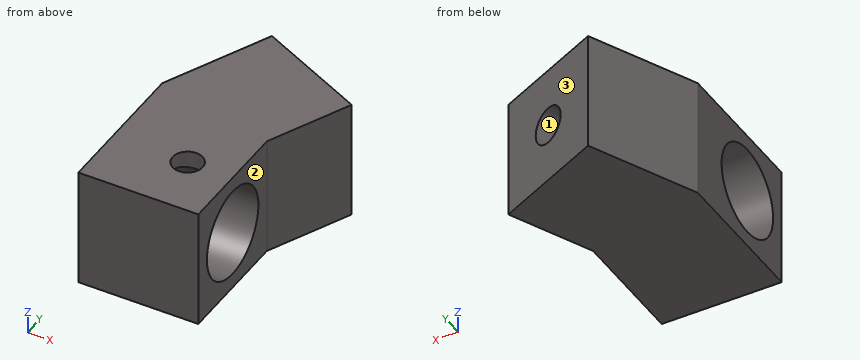
from build123d import *

# Parameters (mm, degrees)
BOSS_EXTRUDE1_DEPTH = 8
CUT_EXTRUDE1_REACH  = 10
SKETCH3_R           = 3
CUT_EXTRUDE2_REACH  = 10
SKETCH4_R           = 1
SKETCH5_R           = 1.25
CUT_EXTRUDE3_DEPTH  = 3


with BuildPart() as part:
    # Sketch2 → Boss-Extrude1 (new body)
    with BuildSketch(Plane.XY):
        Polygon((8, 0), (0, 0), (0, 9.773557301), (3.285247274, 16.818792816), (10.53570957, 13.437846722), (8, 8), align=None)
    extrude(amount=BOSS_EXTRUDE1_DEPTH)

    # Sketch3 → Cut-Extrude1 (cut, up to next)
    with BuildSketch(Plane(origin=(8, 0, 0), x_dir=(0, 0, -1), z_dir=(1, 0, 0)), mode=Mode.PRIVATE) as cut_extrude1_sk1:
        with Locations((-4, 4)):
            Circle(SKETCH3_R)
    cut_extrude1_tool1 = extrude(cut_extrude1_sk1.sketch, amount=-CUT_EXTRUDE1_REACH, mode=Mode.PRIVATE) & part.part
    add(cut_extrude1_tool1.solids().sort_by_distance((8, 4, 4))[0], mode=Mode.SUBTRACT)

    # Sketch4 → Cut-Extrude2 (cut, up to next)
    with BuildSketch(Plane.XY.offset(8), mode=Mode.PRIVATE) as cut_extrude2_sk1:
        with Locations((5, 4)):
            Circle(SKETCH4_R)
    cut_extrude2_tool1 = extrude(cut_extrude2_sk1.sketch, amount=-CUT_EXTRUDE2_REACH, mode=Mode.PRIVATE) & part.part
    add(cut_extrude2_tool1.solids().sort_by_distance((5, 4, 8))[0], mode=Mode.SUBTRACT)

    # Sketch5 → Cut-Extrude3 (cut)
    with BuildSketch(Plane(origin=(7.028736904, 15.073174933, 0), x_dir=(0.906307787, -0.422618262, 0), z_dir=(0.422618262, 0.906307787, 0))):
        with Locations((-0.130483798, -4)):
            Circle(SKETCH5_R)
    extrude(amount=-CUT_EXTRUDE3_DEPTH, mode=Mode.SUBTRACT)


solid = part.part
Work out the finished part from the listing and answer in its coordinate system (mm). Face numbers are marked on the shaded views. Coordinates: 2 decimals unless noted, no trailing zeros. Loops run counter-clockwise (first coordinate to the right, second up) from the corner with the lowest first, then second, coordinate; pieces in that order, holes last. Notation, with made-up numbers: M 5.25,51.5 L 51.25,51.5 A15 cw 51.25,74.5 Z; hole C 12.25,85.25 d8. An arc over 180 degrees is marked long. Answer in a Markdown table with one row per item. Add a question column.
1. Find section C-C, the plane y = 2. Write down the section's boundary in (x, z), then the cut area to 3 significant figures.
2. Find section D-D, the plane z = 5.5. Write down the section's boundary in (x, y), then the cut area to 3 significant figures.
3. The mould has two halves that part along Y. Classify the marked faces 1, 2 and 3: pulls with the +Y half, pulls with the -Y half, needs draft (parallel to the pull), parting line crosses it, or undercut.
4. Consider L1, parallel to X at y = 4, z = 7.4; L2, parallel to X at y = 7, z = 0.75; L3, parallel to Z at x = 2, y = 4. Determine where each line is inside the solid, lowest interval first.
5. Find section B-B, the plane z = 4.5. Write down the section's boundary in (x, y).
6. Flat-ended cylindrical pins translate along their axes: P1, Ø1.5, axis at y = 12.5, z = 6, coming from the -X side; P2, Ø2, axis at x = 8, z = 6, coming from the +Y side; P3, Ø3, axis at x = 7.5, z = 1.5, coming from the +Y side. Find the tip coordinate at first contact, or state that the pin passes through.
7. Find section A-A, the plane y = 4. Write down the section's boundary in (x, z).
Reported:
| question | item | result |
|---|---|---|
| 1 | outline | M 0,0 L 8,0 L 8,1.76 L 0,1.76 Z; M 0,6.24 L 8,6.24 L 8,8 L 0,8 Z |
| 1 | area | 28.2 mm^2 |
| 2 | outline | M 0,0 L 8,0 L 8,1.4 L 0,1.4 Z; M 0,6.6 L 8,6.6 L 8,8 L 10.54,13.44 L 3.29,16.82 L 0,9.77 Z |
| 2 | area | 84.6 mm^2 |
| 3 | face 1 | undercut |
| 3 | face 2 | needs draft |
| 3 | face 3 | pulls with the +Y half |
| 4 | L1 | x = 0 to 4, 6 to 8 |
| 4 | L2 | x = 0 to 8 |
| 4 | L3 | z = 0 to 1, 7 to 8 |
| 5 | outline | M 0,0 L 8,0 L 8,1.04 L 0,1.04 Z; M 0,6.96 L 8,6.96 L 8,8 L 10.54,13.44 L 7.95,14.64 L 6.68,11.93 L 4.6,12.89 L 5.87,15.61 L 3.29,16.82 L 0,9.77 Z |
| 6 | P1 | stops at x = 0.92 |
| 6 | P2 | stops at y = 15.09 |
| 6 | P3 | stops at y = 15.55 |
| 7 | outline | M 0,0 L 8,0 L 8,1 L 0,1 Z; M 0,7 L 4,7 L 4,8 L 0,8 Z; M 6,7 L 8,7 L 8,8 L 6,8 Z |
